Verification items for the finished model (mm, model axes). Coordinates: 2 decimals unless noted, no trailing zeros. Write each loop counter-clockwise with the first axis right and the second up, starting at its lowest first coordinate (ties: lowest second). Pieces come first, ordered by that corner, then holes. Notation, with made-up numbers: (54.5, -39) -> (100.5, -39) arc R23 ccw to (100.5, -18) -> close; hole circle Ø2 at (-30.75, -13.5). An arc over 180 degrees is marked (long way). Answer in a Markdown table with one row per item.
```python
from build123d import *

# Parameters (mm, degrees)
F0_R     = 40
F1_DEPTH = 100
F2_SIZE  = 5
F4_D     = 17.5
F4_DEPTH = 19.5
F4_TIP   = 5.2575304165


with BuildPart() as f1:
    # F0 (on Front) → F1 (new body, symmetric)
    with BuildSketch(Plane.XZ):
        Circle(F0_R)
    extrude(amount=F1_DEPTH, both=True)

    # F2
    f2_edges = [f1.edges().sort_by_distance(p)[0] for p in [
        (-40, 100, 0),
    ]]
    chamfer(f2_edges, length=F2_SIZE)

    # F4
    with Locations(Plane.XZ.offset(100)):
        with Locations((0, 0)):
            Hole(F4_D / 2, depth=F4_DEPTH)
            with Locations((0, 0, -(F4_DEPTH + F4_TIP / 2))):  # 118° drill point
                Cone(0, F4_D / 2, F4_TIP, mode=Mode.SUBTRACT)


solid = f1.part
```
1. Material ranges on probe 1 along Z at (x, y) = (0, -94); probe 2 along X at (y, z) = (-54, -34.5); probe 3 along Z at (x, y) = (-16, 10), recorded low to high. Write a range as from..to.
Findings below:
| item | result |
|---|---|
| probe 1 | z = -40..-8.75, 8.75..40 |
| probe 2 | x = -20.24..20.24 |
| probe 3 | z = -36.66..36.66 |
2. Sectioned sample at A-A, the plane y = 15. Record the cut outline in (x, z), and give its area (3 significant figures).
Findings below:
| item | result |
|---|---|
| outline | circle Ø80 at (0, 0) |
| area | 5,030 mm² |
3. Go/stop test with flat-tipped pins: pin 1 (8 mm diameter, centred on x = -2, y = -62, fed in from +Z); pin 2 (12 mm diameter, centred on x = 21, y = -74, fed in from +Z); pin 3 (10 mm diameter, centred on x = 6.5, y = -67, fed in from -Z). Record where each tip stops, or that it passes through.
Findings below:
| item | result |
|---|---|
| pin 1 | stops at z = 40 |
| pin 2 | stops at z = 37.08 |
| pin 3 | stops at z = -39.97 |
4. Release check for a two-part mould opening along Z. For faces 1 (the face through (6.944, -90.114, -5.324)), 2 (the face through (-1, -100, 9)), 3 (the face through (-0.329, -76.156, -1.483)), 4 (the face through (-8.67, -3.86, -39.05)) record: released by +Z, released by -Z, zero draft, split by the parting line, or undercut.
Findings below:
| item | result |
|---|---|
| face 1 | undercut |
| face 2 | zero draft |
| face 3 | undercut |
| face 4 | split by the parting line |
